Design review of the part built by this model. Coordinates are the model's own, in mm. Face numbers are marked on the shaded views. Coordinates: 2 decimals unless noted, no trailing zeros. Order: outer loops, then holes, each group sorted by start corner. A loop starts at its lowest first (then second) coordinate and runs counter-clockwise, first axis right, second up. Notation, with made-up numbers: (73, 50) -> (85, 50) arc R9 ccw to (85, 65) -> close; hole circle Ø7 at (72, -23). An arc over 180 degrees is marked (long way). Write item = value, one per line.
```python
from build123d import *

# Parameters (mm, degrees)
SKETCH1_R           = 80
BOSS_EXTRUDE1_DEPTH = 19
SKETCH2_R           = 22.5
CUT_EXTRUDE1_DEPTH  = 115.721401665
SKETCH3_R           = 6.580979797
CUT_EXTRUDE2_DEPTH  = 12.899257
CIRPATTERN1_START   = 6.100742756
CIRPATTERN1_DEPTH   = 12.899257244


# Read off the part's stored shape, not the designer's step: CirPattern1
with BuildPart() as part:
    # Sketch1 → Boss-Extrude1 (new body)
    with BuildSketch(Plane(origin=(0, 0, 0), x_dir=(1, 0, 0), z_dir=(0, 1, 0))):
        with Locations(Location((0, 0, 0), (0, 0, 270))):
            Circle(SKETCH1_R)
    extrude(amount=BOSS_EXTRUDE1_DEPTH)

    # Sketch2 → Cut-Extrude1 (cut, through all)
    with BuildSketch(Plane(origin=(0, 0, 0), x_dir=(1, 0, 0), z_dir=(0, 1, 0))):
        with Locations(Location((0, 0, 0), (0, 0, 270))):
            Circle(SKETCH2_R)
    extrude(amount=CUT_EXTRUDE1_DEPTH, mode=Mode.SUBTRACT)

    # Sketch3 → Cut-Extrude2 (cut)
    with BuildSketch(Plane(origin=(0, 19, 0), x_dir=(1, 0, 0), z_dir=(0, 1, 0))):
        with Locations((-21.524179489, 0)):
            Circle(SKETCH3_R)
    extrude(amount=-CUT_EXTRUDE2_DEPTH, mode=Mode.SUBTRACT)

    # CirPattern1 outline → CirPattern1 (cut)
    with BuildSketch(Plane(origin=(0, 0, 0), x_dir=(1, 0, 0), z_dir=(0, 1, 0)).offset(CIRPATTERN1_START)):
        with BuildLine():
            ThreePointArc((-0.389948756, -22.496620634), (-6.952882374, -21.398771617), (-12.907706665, -18.429354537))
            ThreePointArc((-12.907706665, -18.429354537), (-8.684971849, -26.729594881), (-0.389948756, -22.496620634))
        make_face()
        with BuildLine():
            ThreePointArc((-0.389948756, 22.496620634), (-8.684971849, 26.729594881), (-12.907706665, 18.429354537))
            ThreePointArc((-12.907706665, 18.429354537), (-6.952882374, 21.398771617), (-0.389948756, 22.496620634))
        make_face()
        with BuildLine():
            ThreePointArc((21.275056856, -7.322701398), (18.202882373, -13.225168177), (13.538657006, -17.970942281))
            ThreePointArc((13.538657006, -17.970942281), (22.737551492, -16.519798142), (21.275056856, -7.322701398))
        make_face()
        with BuildLine():
            ThreePointArc((21.275056856, 7.322701398), (22.737551492, 16.519798142), (13.538657006, 17.970942281))
            ThreePointArc((13.538657006, 17.970942281), (18.202882373, 13.225168177), (21.275056856, 7.322701398))
        make_face()
    extrude(amount=CIRPATTERN1_DEPTH, mode=Mode.SUBTRACT)


solid = part.part
```
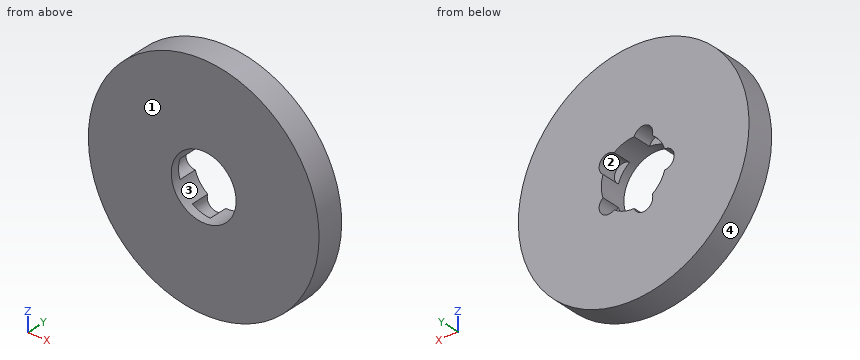
(1) We need section D-D (x = -53). Write out the cut boundary in (y, z).
Report:
outline = (0, -59.92) -> (19, -59.92) -> (19, 59.92) -> (0, 59.92) -> close
(2) We need section C-C (y = 15.5). Write out the cut boundary in (x, z), and give its area (3 significant figures).
Report:
outline = circle Ø160 at (0, 0); hole (-21.52, -6.58) arc R22.5 ccw to (-12.91, -18.43) arc R6.58 ccw to (-0.39, -22.5) arc R22.5 ccw to (13.54, -17.97) arc R6.58 ccw to (21.28, -7.32) arc R22.5 ccw to (21.28, 7.32) arc R6.58 ccw to (13.54, 17.97) arc R22.5 ccw to (-0.39, 22.5) arc R6.58 ccw to (-12.91, 18.43) arc R22.5 ccw to (-21.52, 6.58) arc R6.58 ccw to start
area = 18,200 mm²
(3) Insertion check: pin 1 (2 mm diameter, centred on x = -26, z = 1.5, fed in from +Y); pin 2 (9.5 mm diameter, centred on x = -8.5, z = -23.5, fed in from +Y); pin 3 (5 mm diameter, centred on y = 9, z = 56.5, fed in from +X); pin 4 (6 mm diameter, centred on x = -63, y = 15.5, fed in from -Z) (3 decimals). Each pin has a flat end and moves straight along its axis. Give the tip position at first contact, or say it passes through.
Report:
pin_1 = 6.1
pin_2 = 19
pin_3 = 59.03
pin_4 = -52.915
(4) We need section A-A (z = 0). Write out the cut boundary in (x, y).
Report:
outline = (-80, 0) -> (-22.5, 0) -> (-22.5, 6.1) -> (-28.11, 6.1) -> (-28.11, 19) -> (-80, 19) -> close; (22.5, 0) -> (80, 0) -> (80, 19) -> (22.5, 19) -> close
(5) For L1, parallel to X at y = 5.5, z = 0; L2, parallel to X at y = 11.75, z = 0; L3, parallel to Z at x = -7, y = 3, list the stretches that pass through material, from the lowest coordinate up.
Report:
L1 = -80 to -22.5, 22.5 to 80
L2 = -80 to -28.11, 22.5 to 80
L3 = -79.69 to -21.38, 21.38 to 79.69
(6) We need section B-B (x = 3). Write out the cut boundary in (y, z), and give its area (3 significant figures).
Report:
outline = (0, -79.94) -> (19, -79.94) -> (19, -22.3) -> (0, -22.3) -> close; (0, 22.3) -> (19, 22.3) -> (19, 79.94) -> (0, 79.94) -> close
area = 2,190 mm²
(7) The part is to be moulded in two halves that separate along Z. For the marked faces 1, 2, 3 and 4, say which applies: released by +Z, released by -Z, zero draft, split by the parting line, or undercut.
Report:
face_1 = zero draft
face_2 = undercut
face_3 = undercut
face_4 = split by the parting line
